Autodesk Inventor part; units mm, degrees
ref_plane "YZ Plane" through (0, 0, 0) normal (1, 0, 0) x (0, 1, 0)
ref_plane "XZ Plane" through (0, 0, 0) normal (0, 1, 0) x (-1, 0, 0)
ref_plane "XY Plane" through (0, 0, 0) normal (0, 0, 1) x (1, 0, 0)
sketch "Sketch1" plane through (0, 0, 0) normal (0, 1, 0) x (-1, 0, 0)
  line L0 (0, 0) -> (-9.6, 0)
  circle A0 centre (0, 0) radius 1.45
  circle A1 centre (-9.6, 0) radius 1.45
  line L1 (0, 0) -> (4, 0)
  line L2 (4, 0) -> (4, -4)
  line L3 (-9.6, 0) -> (-13.6, 0)
  line L4 (-13.6, 0) -> (-13.6, 4)
  line L5 (4, -4) -> (-13.6, -4)
  line L6 (-13.6, -4) -> (-13.6, 4)
  line L7 (-13.6, 4) -> (4, 4)
  line L8 (4, 4) -> (4, -4)
  line L9 (4, 4) -> (4, 10.4)
  line L10 (4, 10.4) -> (-13.6, 10.4)
  line L11 (-13.6, 10.4) -> (-13.6, 4)
  dimension "d0" = 9.6
  dimension "d1" = 2.9
  dimension "d4" = 4
  dimension "d7" = 6.4
extrude "Extrusion1" add sketch "Sketch1" along normal blind 6.4 contours A1 L3 L4 L7 L8 L1 A0 L0 | L0 A0 L1 L2 L5 L6 L3 A1
extrude "Extrusion2" add sketch "Sketch1" against normal blind 3.2 contours A1 L3 L4 L7 L8 L1 A0 L0 | L0 A0 L1 L2 L5 L6 L3 A1 | L11 L10 L9 L7
properties part number "deadbolt enclosure wall holder bracket"
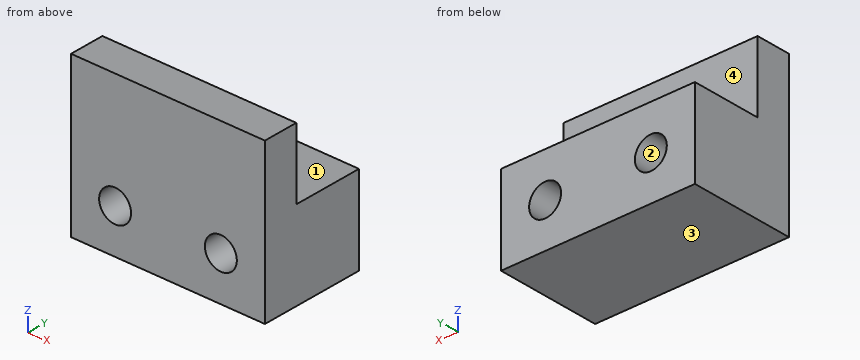
The listing builds one solid part. Answer for the finished solid, in the listing's coordinates (mm). Face numbers are marked on the shaded views. Coordinates: 2 decimals unless noted, no trailing zeros. Write each loop counter-clockwise with the first axis right and the second up, starting at its lowest first coordinate (ties: lowest second). Pieces come first, ordered by that corner, then holes. Notation, with made-up numbers: (84.5, 72.25) - (143.5, 72.25) arc R21 ccw to (143.5, 101.25) - close; hole circle Ø5 at (-30.75, 53.5). An arc over 180 degrees is marked (long way). Return JSON: item names as keys, results as strings. Group by question number.
1. A cutting plane is placed at B-B, the plane x = 0. Determine the outline of the cut face in (y, z).
2. A cutting plane is placed at D-D, the plane x = 7.75. Determine the outline of the cut face in (y, z).
3. Determine the mould class of the marked faces 1, 2, 3 and 4 for opening direction Z: released by +Z, released by -Z, zero draft, split by the parting line, or undercut.
4. A cutting plane is placed at A-A, the plane z = 0. Determine the outline of the cut face in (x, y).
5. Given pin 1 (5 mm diameter, centred on x = 1, z = 7.5, fed in from +Y), flat-ended and moving along its own axis, determine where the tip first touches the part or whether it passes through.
6. A cutting plane is placed at C-C, the plane y = -2. Determine the outline of the cut face in (x, z).
7. Straight lines are drawn through the part: L1, parallel to X at y = 0.75, z = 0; L2, parallel to X at y = -1.5, z = -1.25; L3, parallel to Z at x = 9.6, y = 0.5. For each, find the intervals that lie inside material, in ascending order.
Ans:
{
 "1": {"outline": "(-3.2, -4) - (6.4, -4) - (6.4, -1.45) - (-3.2, -1.45) - close; (-3.2, 1.45) - (6.4, 1.45) - (6.4, 4) - (0, 4) - (0, 10.4) - (-3.2, 10.4) - close"},
 "2": {"outline": "(-3.2, -4) - (6.4, -4) - (6.4, 4) - (0, 4) - (0, 10.4) - (-3.2, 10.4) - close"},
 "3": {"face 1": "released by +Z", "face 2": "undercut", "face 3": "released by -Z", "face 4": "zero draft"},
 "4": {"outline": "(-4, -3.2) - (-1.45, -3.2) - (-1.45, 6.4) - (-4, 6.4) - close; (1.45, -3.2) - (8.15, -3.2) - (8.15, 6.4) - (1.45, 6.4) - close; (11.05, -3.2) - (13.6, -3.2) - (13.6, 6.4) - (11.05, 6.4) - close"},
 "5": {"pin 1": "y = 0"},
 "6": {"outline": "(-4, -4) - (13.6, -4) - (13.6, 10.4) - (-4, 10.4) - close; hole circle Ø2.9 at (0, 0); hole circle Ø2.9 at (9.6, 0)"},
 "7": {"L1": "-4 to -1.45, 1.45 to 8.15, 11.05 to 13.6", "L2": "-4 to -0.73, 0.73 to 8.87, 10.33 to 13.6", "L3": "-4 to -1.45, 1.45 to 4"}
}
